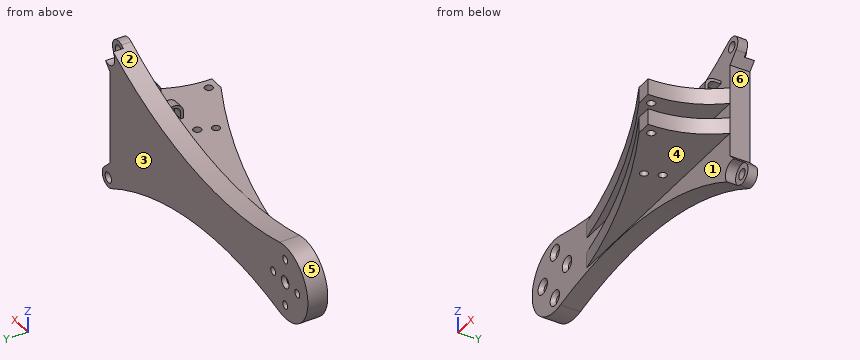
Autodesk Inventor part; units mm, degrees
ref_plane "YZ Plane" through (0, 0, 0) normal (1, 0, 0) x (0, 1, 0)
ref_plane "XZ Plane" through (0, 0, 0) normal (0, 1, 0) x (-1, 0, 0)
ref_plane "XY Plane" through (0, 0, 0) normal (0, 0, 1) x (1, 0, 0)
sketch "Sketch1" plane through (0, 0, 0) normal (0, 1, 0) x (-1, 0, 0)
  line L0 (0, 0) -> (105.9629, 0) construction
  line L1 (105.9629, 0) -> (105.9629, -9.5) construction
  circle A0 centre (105.9629, -9.5) radius 1.6
  circle A1 centre (113.9629, 0) radius 1.6
  circle A2 centre (105.9629, -9.5) radius 1.6
  circle A3 centre (97.9629, 0) radius 1.6
  circle A4 centre (105.9629, 9.5) radius 1.6
  circle A5 centre (105.9629, 0) radius 15
  circle A6 centre (105.9629, 0) radius 2.5
  line L2 (3, -40) -> (-37, 0) construction
  line L3 (-7.5, -16.5) -> (-14, -23)
  circle A7 centre (-11.1716, -25.8284) radius 4
  circle A8 centre (-11.1716, -25.8284) radius 2.1
  arc A9 (102.2211, -14.5258) -> (-9.1982, -29.3078) centre (64.8022, -159.7836) ccw
  line L4 (3, 40) -> (-37, 0) construction
  line L5 (-7.5, 16.5) -> (-14, 23)
  circle A10 centre (-11.1716, 25.8284) radius 4
  circle A11 centre (-11.1716, 25.8284) radius 2.1
  arc A12 (-9.1982, 29.3078) -> (102.2211, 14.5258) centre (64.8022, 159.7836) ccw
  line L6 (-10, 19) -> (-10, -19)
  arc A13 (-12.9845, 21.9845) -> (-6.9989, 26.6354) centre (-11.1716, 25.8284) ccw
  arc A14 (-7.9621, -28.6144) -> (-12.9845, -21.9845) centre (-11.1716, -25.8284) ccw
  arc A15 (-6.9989, 26.6354) -> (-7.9621, 28.6144) centre (-11.1716, 25.8284) ccw
  point P0 (-16.1526, 27.519)
  point P1 (-14, -23)
  point P2 (102.2211, 14.5258)
  point P3 (-14, 23)
  point P4 (-10, 0)
  point P5 (-12.9845, -21.9845)
  dimension "d5" = 30
  dimension "d67" = 8
  dimension "d1" = 9.5
  dimension "d2" = 3.2
  dimension "d3" = 3.2
  dimension "d4" = 8
  dimension "d55" = 5
  dimension "d68" = 4
  dimension "d69" = 4.2
  dimension "d70" = 150
  dimension "d82" = 10
  dimension "d84" = 38
  dimension "d85" = 105.963
  dimension "d86" = 4.25
extrude "Extrusion1" add sketch "Sketch1" along normal blind 8 contours A5 | A5 A9 A14 L3 L6 L5 A13 A15 A12 | A6
extrude "Extrusion2" add sketch "Sketch1" along normal blind 3.9 contours A15 A13 L5 A10 A12 | A10
extrude "Extrusion3" add sketch "Sketch1" against normal blind 3.9 from surface at 8 contours A9 A7 L3 A14 | A7
extrude "Extrusion9" cut sketch "Sketch1" against normal blind 2 from surface at 8 contours A6
sketch "Sketch2" plane through (0, 0, 0) normal (0, 0, 1) x (1, 0, 0)
  line L0 (0, 0) -> (-3, 0)
  line L1 (0, 0) -> (0, -30)
  line L2 (-98.8932, 0) -> (-6, 0)
  arc A0 (0, -30) -> (-85, 0) centre (-137.8451, -285.1445) ccw
  line L3 (-6, -26.8484) -> (0, -26.8484)
  line L4 (0, 0) -> (-85, 0)
  line L5 (0, -23.1484) -> (-13.5147, -23.1484) construction
  circle A1 centre (-4, -23.1484) radius 1.6
  arc A2 (10, 0) -> (0, -26.8484) centre (39.9981, -26.4597) ccw
  line L6 (10, 0) -> (0, 0)
  line L7 (12.9845, 8) -> (10, 8)
  point P0 (0, -15)
  point P1 (-3, 0)
  point P2 (-6, 0)
  point P3 (-85, 0)
  point P4 (12.622, 8)
  point P5 (0, 8)
  point P6 (0, -26.0709)
  point P7 (14, 8)
  point P8 (12.7592, 8)
  dimension "d16" = 290
  dimension "d17" = 85
  dimension "d18" = 6
  dimension "d19" = 30
  dimension "d63" = 3.7
  dimension "d64" = 3.2
  dimension "d65" = 4
  dimension "d79" = 10
  dimension "d80" = 40
extrude "Extrusion4" add sketch "Sketch2" along normal mid plane 19 contours L6 A2 L3 A0 L2 L4 L0
extrude "Extrusion11" cut sketch "Sketch2" along normal mid plane 6 contours L6 A2 L3 A0 L2 L4 L0 | A1
sketch "Sketch9" plane through (0, 0, 9.5) normal (0, 0, 1) x (1, 0, 0)
  circle A0 centre (-26, -12.7093) radius 1.6
  arc A1 (-6, -26.8484) -> (-85, 0) centre (-137.8451, -285.1445) ccw
  line L0 (0, -26.8484) -> (0, 0)
  line L1 (-137.8451, -285.1445) -> (-26, -12.7093) construction
  line L2 (-26, -12.7093) -> (-21.4388, -1.5991) construction
  circle A2 centre (-23.5314, -6.6963) radius 1.6
  line L3 (0, 0) -> (0, -45) construction
  point P0 (0, -13.4242)
  dimension "d71" = 3.2
  dimension "d72" = 294.5
  dimension "d73" = 26
  dimension "d75" = 3.2
  dimension "d76" = 6.5
extrude "Extrusion12" cut sketch "Sketch9" against normal through all
sketch "Sketch10" plane through (10, 0, -19) normal (1, 0, 0) x (0, 0, -1)
  line L0 (-38, 0) -> (-28.5, 0)
  line L1 (-28.5, 0) -> (-28.5, -7)
  line L2 (-28.5, -26.8484) -> (-28.5, 0)
  line L3 (-28.5, 0) -> (-37.25, 0)
  circle A0 centre (-31.1, -2.6) radius 2.6
  arc A1 (-34.85, -2.6) -> (-31.1, -6.35) centre (-31.1, -2.6) ccw
  line L4 (-34.85, -2.6) -> (-34.85, 0)
  line L5 (-31.1, -6.35) -> (-28.5, -6.35)
  line L6 (-31.1, -5.2) -> (-28.5, -5.2)
  line L7 (-33.7, -2.6) -> (-33.7, 0)
  arc A2 (-28.5, -5.3023) -> (-33.8023, 0) centre (-31.1, -2.6) ccw
  arc A3 (-31.1, -6.35) -> (-28.5, -5.3023) centre (-31.1, -2.6) ccw construction
  point P0 (-19, 0)
  point P1 (-33.7, 0)
  point P2 (-34.85, 0)
  point P3 (-32.4068, -0.3523)
  point P4 (-31.1, 0)
  point P5 (-28.5, -2.6)
  point P6 (-31.1, 0)
  dimension "d101" = 5.2
  dimension "d102" = 7.5
extrude "Extrusion16" add sketch "Sketch10" against normal blind 25 contours L0 L7 A0 L6 L1 L5 A1 L4
extrude "Extrusion17" cut sketch "Sketch10" against normal blind 21 contours L0 L7 A0 L6 L1 L5 A1 L4 | L0 A0 L7 | L0 L1 A0 | L6 A0 L1
extrude "Extrusion18" add sketch "Sketch10" against normal blind 10 contours L0 L7 A0 L6 L1 L5 A1 L4
extrude "Extrusion19" cut sketch "Sketch10" against normal blind 6 contours L0 L7 A0 L6 L1 L5 A1 L4 | L0 A0 L7 | L0 L1 A0 | L6 A0 L1
chamfer "Chamfer1" distance 1.5 angle 45 4 edges at (-104.3629, 0, 9.5) (-96.3629, 0, 0) (-112.3629, 0, 0) (-104.3629, 0, -9.5)
properties part number "brat"
Model file for the job. Use its own axes, mm. Face numbers are marked on the shaded views. A direction names the side the tool comes from. Coordinates: 2 decimals unless noted, no trailing zeros. Write each loop counter-clockwise with the first axis right and the second up, starting at its lowest first coordinate (ties: lowest second). Pieces come first, ordered by that corner, then holes. Notation, with made-up numbers: (8, 87) - (34, 87) arc R18 ccw to (34, 94) - close; hole circle Ø8 at (-30.75, -36). An arc over 180 degrees is marked (long way). One line per item, written item: value. Start each with the question number.
1. Slice it at B-B (y = -17). Write the cut outline in (x, z).
2. Slice it at C-C (x = -4). Write the cut outline in (y, z).
3. Probe line 1 (Z direction, x = -13.5, y = -2); line 2 (Z direction, x = -2, y = -15.5); line 3 (Y direction, x = -4, z = 8). List the from-to ranges inside material, lowest first. Write a range as from..to.
4. Tool access for the marked faces 4, 5 and 6: list every direction of +Z, -Z, +X, -X, +Y, -Y with a clear straight run to the whole face (end or side of a thin tool).
5. Flat gauge pins, fed straight in: pin 1 (1.3 mm diameter, centred on x = -12, z = 10.5, fed in from -Y); pin 2 (1.5 mm diameter, centred on x = -1, y = 1.5, fed in from -Z); pin 3 (5 mm diameter, centred on x = -4, y = -23.15, fed in from +Z); pin 4 (5 mm diameter, centred on x = -113.96, z = 0, fed in from +Y). Where does each tip first touch, or does it go through?
6. Slice it at A-A (z = 0). Write the cut outline in (x, y).
7. Mould opens along Z. For the marked faces 1, 2 and 3 say: released by +Z, released by -Z, zero draft, split by the parting line, or undercut.
Answers below:
1. outline: (-27.4, -9.5) - (1.13, -9.5) - (1.13, -3) - (-27.4, -3) - close; (-27.4, 3) - (1.13, 3) - (1.13, 9.5) - (-27.4, 9.5) - close
2. outline: (-26.85, -9.5) - (-24.75, -9.5) - (-24.75, -3) - (-26.85, -3) - close; (-26.85, 3) - (-24.75, 3) - (-24.75, 9.5) - (-26.85, 9.5) - close; (-21.55, -9.5) - (0, -9.5) - (0, -22.66) - (8, -22.66) - (8, 22.66) - (0, 22.66) - (0, 9.5) - (-21.55, 9.5) - (-21.55, 3) - (0, 3) - (0, -3) - (-21.55, -3) - close
3. line 1: z = -9.5..-3, 3..9.5, 14.7..15.85
3. line 2: z = -9.5..-3, 3..9.5
3. line 3: y = -26.85..-24.75, -21.55..8
4. face 4: -Z, +X, -X, -Y
4. face 5: +Y, -Y
4. face 6: +X, +Y, -Y
5. pin 1: stops at y = -6.35
5. pin 2: stops at z = -24.38
5. pin 3: stops at z = 9.5
5. pin 4: stops at y = 8
6. outline: (-120.96, 0) - (-117.06, 0) - (-115.56, 1.5) - (-115.56, 8) - (-120.96, 8) - close; (-112.36, 1.5) - (-110.86, 0) - (-101.06, 0) - (-99.56, 1.5) - (-99.56, 8) - (-103.46, 8) - (-103.46, 6) - (-108.46, 6) - (-108.46, 8) - (-112.36, 8) - close; (-96.36, 1.5) - (-94.86, 0) - (10, 0) - (10, 8) - (-96.36, 8) - close
7. face 1: undercut
7. face 2: released by +Z
7. face 3: zero draft
